from build123d import *
from OCP.BRepFilletAPI import BRepFilletAPI_MakeChamfer

# Parameters (mm, degrees)
BOSS_EXTRUDE1_DEPTH = 0.255
SKETCH2_R           = 0.7
CUT_EXTRUDE1_DEPTH  = 9.625827497
CHAMFER1_SIZE       = 0.4
CHAMFER1_SIZE2      = 0.027970725


with BuildPart() as part:
    # Sketch1 → Boss-Extrude1 (new, symmetric)
    with BuildSketch(Plane(origin=(0, 0, 0), x_dir=(1, 0, 0), z_dir=(0, 1, 0))):
        Polygon((0, 1.98), (-1.27, 1.98), (-1.27, 1.46), (-7.78, 1.46), (-8.38, 0.86), (-8.38, 0), (4.19, 0), (4.19, 0.38), (1.4, 0.635), (0, 0.635), align=None)
    boss_extrude1 = extrude(amount=BOSS_EXTRUDE1_DEPTH, both=True)

    # Mirror1: Boss-Extrude1 across plane
    add(boss_extrude1.mirror(Plane(origin=(-8.38, 0.255, 0), x_dir=(1, 0, 0), z_dir=(0, 0, -1))))

    # Sketch2 → Cut-Extrude1 (cut, through all)
    with BuildSketch(Plane(origin=(0, 0.255, 0), x_dir=(1, 0, 0), z_dir=(0, 1, 0))):
        with Locations(Location((-6.88, 0, 0), (0, 0, 270))):
            Circle(SKETCH2_R)
    extrude(amount=-CUT_EXTRUDE1_DEPTH, mode=Mode.SUBTRACT)

    # Chamfer1: one chamfer whose edges measure the first distance from different faces: ONE call of the kernel's chamfer builder (chamfer() names one face for all edges)
    chamfer1_edges_1 = [part.edges().sort_by_distance(p)[0] for p in [
        (-8.38, -0.255, 0),
    ]]
    chamfer1_side_1 = [part.faces().sort_by_distance(p)[0] for p in [
        (-2.842081645, -0.255, 0),
    ]]
    chamfer1_edges_2 = [part.edges().sort_by_distance(p)[0] for p in [
        (-8.38, 0.255, 0),
    ]]
    chamfer1_side_2 = [part.faces().sort_by_distance(p)[0] for p in [
        (-2.842081645, 0.255, 0),
    ]]
    chamfer1 = BRepFilletAPI_MakeChamfer(part.part.solid().wrapped)
    for e in chamfer1_edges_1:
        chamfer1.Add(CHAMFER1_SIZE, CHAMFER1_SIZE2, e.wrapped, chamfer1_side_1[0].wrapped)  # the first distance lies on this face
    for e in chamfer1_edges_2:
        chamfer1.Add(CHAMFER1_SIZE, CHAMFER1_SIZE2, e.wrapped, chamfer1_side_2[0].wrapped)  # the first distance lies on this face
    add(Compound.cast(chamfer1.Shape()), mode=Mode.REPLACE)


solid = part.part
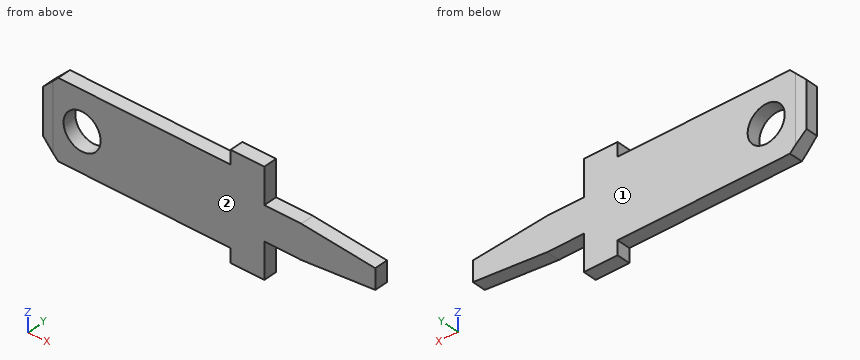
CAD build for the part. Positions are in the model's coordinates, mm. Face numbers are marked on the shaded views. Round coordinates to 2 decimals unless told otherwise and drop trailing zeros. Write each loop counter-clockwise with the first axis right and the second up, starting at its lowest first coordinate (ties: lowest second). Pieces come first, ordered by that corner, then holes.
(1) Slice it at C-C, the plane z = 0. Write the cut outline in (x, y) (3 decimals).
(2) Drop a flat-ended pin along its axis: P1, Ø0.8, axis at x = -6.88, z = 0, coming from the +Y side. Give the stop position or say it passes through.
(3) Slice it at B-B, the plane x = -6.88. Write the cut outline in (y, z) (3 decimals), and give its area (3 significant figures).
(4) Slice it at D-D, the plane x = 0.5. Write the cut outline in (y, z) (3 decimals).
(5) Probe line 1 along X through (y, z) = (0, 0); line 2 along Z through (x, y) = (-1.5, -0.05); line 3 along Z through (x, y) = (0.5, 0.05) (3 decimals). List the from-to ranges inside material, lowest first.
(6) Slice it at A-A, the plane y = 0.15. Write the cut outline in (x, z) (3 decimals).
(7) Mould opens along Y. For the marked faces 1 and 2 say: pulls with the +Y half, pulls with the -Y half, needs draft (parallel to the pull), parting line crosses it, or undercut.
From the geometry:
1. outline: (-8.38, -0.227) - (-7.98, -0.255) - (-7.58, -0.255) - (-7.58, 0.255) - (-7.98, 0.255) - (-8.38, 0.227) - close; (-6.18, -0.255) - (4.19, -0.255) - (4.19, 0.255) - (-6.18, 0.255) - close
2. P1: passes through
3. outline: (-0.255, -1.46) - (0.255, -1.46) - (0.255, -0.7) - (-0.255, -0.7) - close; (-0.255, 0.7) - (0.255, 0.7) - (0.255, 1.46) - (-0.255, 1.46) - close
3. area: 0.775 mm2
4. outline: (-0.255, -0.635) - (0.255, -0.635) - (0.255, 0.635) - (-0.255, 0.635) - close
5. line 1: x = -8.38 to -7.58, -6.18 to 4.19
5. line 2: z = -1.46 to 1.46
5. line 3: z = -0.635 to 0.635
6. outline: (-8.38, -0.86) - (-7.78, -1.46) - (-1.27, -1.46) - (-1.27, -1.98) - (0, -1.98) - (0, -0.635) - (1.4, -0.635) - (4.19, -0.38) - (4.19, 0.38) - (1.4, 0.635) - (0, 0.635) - (0, 1.98) - (-1.27, 1.98) - (-1.27, 1.46) - (-7.78, 1.46) - (-8.38, 0.86) - close; hole circle Ø1.4 at (-6.88, 0)
7. face 1: pulls with the +Y half
7. face 2: pulls with the -Y half
